CAD build for the part. Positions are in the model's coordinates, mm. A direction names the side the tool comes from. Give positions to 0.01 mm unless a question says otherwise; leave off trailing zeros. Loops run counter-clockwise (first coordinate to the right, second up) from the corner with the lowest first, then second, coordinate; pieces in that order, holes last.
```python
from build123d import *

# Parameters (mm, degrees)
BOSS_EXTRUDE1_DEPTH       = 3.175
SKETCH2_R                 = 3.302
BOSS_EXTRUDE2_DEPTH       = 3.175
BOSS_EXTRUDE3_DEPTH       = 3.175
BOSS_EXTRUDE4_DEPTH       = 3.175
SKETCH10_R                = 3.302
CUT_EXTRUDE2_DEPTH        = 3.175
BOSS_EXTRUDE6_DEPTH       = 3.175
F_6_CLEARANCE_HOLE1_D     = 3.7973
F_6_CLEARANCE_HOLE1_DEPTH = 25.4
F_6_CLEARANCE_HOLE1_TIP   = 1.140824014
CUT_EXTRUDE8_DEPTH        = 4.7625
SKETCH4_R                 = 25.4
BOSS_EXTRUDE7_DEPTH       = 3.175
CUT_EXTRUDE9_DEPTH        = 3.175
SKETCH19_R                = 9.525
CUT_EXTRUDE10_DEPTH       = 3.175
CUT_EXTRUDE12_DEPTH       = 4.175


with BuildPart() as part:
    # Sketch1 → Boss-Extrude1 (new body)
    with BuildSketch(Plane.XY):
        Polygon((-150.669615327, -62.417005507), (-62.404018861, -150.674994572), (62.417005507, -150.669615327), (150.674994572, -62.404018861), (150.669615327, 62.417005507), (62.404018861, 150.674994572), (-62.417005507, 150.669615327), (-150.674994572, 62.404018861), align=None)
        Polygon((-137.969842044, -57.155945955), (-57.144053939, -137.974767879), (57.155945955, -137.969842044), (137.974767879, -57.144053939), (137.969842044, 57.155945955), (57.144053939, 137.974767879), (-57.155945955, 137.969842044), (-137.974767879, 57.144053939), align=None, mode=Mode.SUBTRACT)
    extrude(amount=BOSS_EXTRUDE1_DEPTH)

    # Sketch2 → Boss-Extrude2 (add)
    with BuildSketch(Plane.XY.offset(3.175)):
        with BuildLine():
            Line((-104.300258744, 90.821465649), (-90.83045509, 104.292430334))
            ThreePointArc((-90.83045509, 104.292430334), (-90.829874575, 90.822046164), (-104.300258744, 90.821465649))
        make_face()
        with Locations((-94.197615746, 94.189497078)):
            Circle(SKETCH2_R, mode=Mode.SUBTRACT)
        with BuildLine():
            Line((104.292430334, 90.83045509), (90.821465649, 104.300258744))
            ThreePointArc((90.821465649, 104.300258744), (90.822046164, 90.829874575), (104.292430334, 90.83045509))
        make_face()
        with Locations((94.189497078, 94.197615746)):
            Circle(SKETCH2_R, mode=Mode.SUBTRACT)
        with BuildLine():
            Line((104.300258744, -90.821465649), (90.83045509, -104.292430334))
            ThreePointArc((90.83045509, -104.292430334), (90.829874575, -90.822046164), (104.300258744, -90.821465649))
        make_face()
        with Locations((94.197615746, -94.189497078)):
            Circle(SKETCH2_R, mode=Mode.SUBTRACT)
        with BuildLine():
            Line((-104.292430334, -90.83045509), (-90.821465649, -104.300258744))
            ThreePointArc((-90.821465649, -104.300258744), (-90.822046164, -90.829874575), (-104.292430334, -90.83045509))
        make_face()
        with Locations((-94.189497078, -94.197615746)):
            Circle(SKETCH2_R, mode=Mode.SUBTRACT)
    extrude(amount=-BOSS_EXTRUDE2_DEPTH)

    # Sketch5 → Boss-Extrude3 (add)
    with BuildSketch(Plane.XY.offset(3.175)):
        with BuildLine():
            Line((137.970389359, 44.455945967), (137.969842044, 57.155945955))
            Line((137.969842044, 57.155945955), (128.989198921, 66.135815058))
            ThreePointArc((128.989198921, 66.135815058), (126.236781441, 52.295360716), (137.970389359, 44.455945967))
        make_face()
        with BuildLine():
            Line((128.994898776, -66.124697061), (137.974767879, -57.144053939))
            Line((137.974767879, -57.144053939), (137.974220564, -44.44405395))
            ThreePointArc((137.974220564, -44.44405395), (126.241288378, -52.284480005), (128.994898776, -66.124697061))
        make_face()
        with BuildLine():
            Line((-137.969842044, -57.155945955), (-137.970389359, -44.455945967))
            ThreePointArc((-137.970389359, -44.455945967), (-126.236781441, -52.295360716), (-128.989198921, -66.135815058))
            Line((-128.989198921, -66.135815058), (-137.969842044, -57.155945955))
        make_face()
        with BuildLine():
            Line((-137.974220564, 44.44405395), (-137.974767879, 57.144053939))
            Line((-137.974767879, 57.144053939), (-128.994898776, 66.124697061))
            ThreePointArc((-128.994898776, 66.124697061), (-126.241288378, 52.284480005), (-137.974220564, 44.44405395))
        make_face()
    extrude(amount=-BOSS_EXTRUDE3_DEPTH)

    # Sketch9 → Boss-Extrude4 (add)
    with BuildSketch(Plane(origin=(0, 0, 0), x_dir=(-1, 0, 0), z_dir=(0, 0, -1))):
        Polygon((-57.144053939, 137.974767879), (-137.969842044, 57.155945955), (-137.974767879, -57.144053939), (-57.155945955, -137.969842044), (57.144053939, -137.974767879), (137.969842044, -57.155945955), (137.974767879, 57.144053939), (57.155945955, 137.969842044), align=None)
        Polygon((-49.254106555, 118.924427839), (-118.92018212, 49.264356627), (-118.924427839, -49.254106555), (-49.264356627, -118.92018212), (49.254106555, -118.924427839), (118.92018212, -49.264356627), (118.924427839, 49.254106555), (49.264356627, 118.92018212), align=None, mode=Mode.SUBTRACT)
    extrude(amount=-BOSS_EXTRUDE4_DEPTH)

    # Sketch10 → Cut-Extrude2 (cut)
    with BuildSketch(Plane.XY):
        with Locations((-94.197615746, 94.189497078)):
            Circle(SKETCH10_R)
        with Locations((94.189497078, 94.197615746)):
            Circle(SKETCH10_R)
        with Locations((-94.189497078, -94.197615746)):
            Circle(SKETCH10_R)
        with Locations((94.197615746, -94.189497078)):
            Circle(SKETCH10_R)
    extrude(amount=CUT_EXTRUDE2_DEPTH, mode=Mode.SUBTRACT)

    # Sketch12 → Boss-Extrude6 (add)
    with BuildSketch(Plane(origin=(0, 0, 0), x_dir=(-1, 0, 0), z_dir=(0, 0, -1))):
        Polygon((6.35, 150.672031572), (-6.35, 150.672031572), (-6.35, 6.35), (-150.672578887, 6.35), (-150.672578887, -6.35), (-6.35, -6.35), (-6.35, -150.672031572), (6.35, -150.672031572), (6.35, -6.35), (150.672578887, -6.35), (150.672578887, 6.35), (6.35, 6.35), align=None)
    extrude(amount=-BOSS_EXTRUDE6_DEPTH)

    # #6 Clearance Hole1
    with Locations(Plane(origin=(0, 0, 0), x_dir=(-1, 0, 0), z_dir=(0, 0, -1))):
        with Locations((-0.418811464, 60.325), (-0.418811464, -37.9222), (-0.418811464, -60.52312), (37.9222, 0), (60.52312, 0), (-60.325, 0)):
            Hole(F_6_CLEARANCE_HOLE1_D / 2, depth=F_6_CLEARANCE_HOLE1_DEPTH)
            with Locations((0, 0, -(F_6_CLEARANCE_HOLE1_DEPTH + F_6_CLEARANCE_HOLE1_TIP / 2))):  # 118° drill point
                Cone(0, F_6_CLEARANCE_HOLE1_D / 2, F_6_CLEARANCE_HOLE1_TIP, mode=Mode.SUBTRACT)

    # Sketch17 → Cut-Extrude8 (cut)
    with BuildSketch(Plane(origin=(0, 0, 0), x_dir=(-1, 0, 0), z_dir=(0, 0, -1))):
        Polygon((-73.383632924, 150.675467746), (-61.318869739, 134.799947792), (60.965361784, 134.794677872), (72.666366941, 150.669173624), align=None)
        Polygon((-61.147982987, -134.794670002), (61.136248536, -134.799939922), (73.018390518, -150.675452006), (-73.031609347, -150.669157884), align=None)
    extrude(amount=-CUT_EXTRUDE8_DEPTH, mode=Mode.SUBTRACT)

    # Sketch4 → Boss-Extrude7 (add)
    with BuildSketch(Plane.XY.offset(3.175)):
        Circle(SKETCH4_R)
    extrude(amount=-BOSS_EXTRUDE7_DEPTH)

    # Sketch18 → Cut-Extrude9 (cut)
    with BuildSketch(Plane.XY.offset(3.175)):
        with BuildLine():
            ThreePointArc((109.296804613, 81.790472735), (103.174175191, 89.389946316), (96.524263045, 96.532582958))
            ThreePointArc((96.524263045, 96.532582958), (91.854529866, 96.532381713), (91.854731111, 91.862648534))
            ThreePointArc((91.854731111, 91.862648534), (98.182941997, 85.065549572), (104.009378392, 77.833713966))
            ThreePointArc((104.009378392, 77.833713966), (108.631470887, 77.16838024), (109.296804613, 81.790472735))
        make_face()
        with BuildLine():
            ThreePointArc((81.790472735, -109.296804613), (89.389946316, -103.174175191), (96.532582958, -96.524263045))
            ThreePointArc((96.532582958, -96.524263045), (96.532381713, -91.854529866), (91.862648534, -91.854731111))
            ThreePointArc((91.862648534, -91.854731111), (85.065549572, -98.182941997), (77.833713966, -104.009378392))
            ThreePointArc((77.833713966, -104.009378392), (77.16838024, -108.631470887), (81.790472735, -109.296804613))
        make_face()
        with BuildLine():
            ThreePointArc((-109.296804613, -81.790472735), (-103.174175191, -89.389946316), (-96.524263045, -96.532582958))
            ThreePointArc((-96.524263045, -96.532582958), (-91.854529866, -96.532381713), (-91.854731111, -91.862648534))
            ThreePointArc((-91.854731111, -91.862648534), (-98.182941997, -85.065549572), (-104.009378392, -77.833713966))
            ThreePointArc((-104.009378392, -77.833713966), (-108.631470887, -77.16838024), (-109.296804613, -81.790472735))
        make_face()
        with BuildLine():
            ThreePointArc((-81.790472735, 109.296804613), (-89.389946316, 103.174175191), (-96.532582958, 96.524263045))
            ThreePointArc((-96.532582958, 96.524263045), (-96.532381713, 91.854529866), (-91.862648534, 91.854731111))
            ThreePointArc((-91.862648534, 91.854731111), (-85.065549572, 98.182941997), (-77.833713966, 104.009378392))
            ThreePointArc((-77.833713966, 104.009378392), (-77.16838024, 108.631470887), (-81.790472735, 109.296804613))
        make_face()
    extrude(amount=-CUT_EXTRUDE9_DEPTH, mode=Mode.SUBTRACT)

    # Sketch19 → Cut-Extrude10 (cut)
    with BuildSketch(Plane.XY.offset(3.175)):
        with Locations((-79.81209335, 106.653091503)):
            Circle(SKETCH19_R)
        with Locations((106.653091503, 79.81209335)):
            Circle(SKETCH19_R)
        with Locations((79.81209335, -106.653091503)):
            Circle(SKETCH19_R)
        with Locations((-106.653091503, -79.81209335)):
            Circle(SKETCH19_R)
    extrude(amount=-CUT_EXTRUDE10_DEPTH, mode=Mode.SUBTRACT)

    # Sketch22 → Cut-Extrude12 (cut, through all)
    with BuildSketch(Plane.XY.offset(3.175)):
        with BuildLine():
            Line((-137.97442785, 49.253969726), (-137.970182132, -49.264493456))
            ThreePointArc((-137.970182132, -49.264493456), (-134.795045306, -52.439356624), (-131.620182138, -49.264219798))
            Line((-131.620182138, -49.264219798), (-131.624427856, 49.254243384))
            ThreePointArc((-131.624427856, 49.254243384), (-134.799564682, 52.429106552), (-137.97442785, 49.253969726))
        make_face()
        with BuildLine():
            Line((131.869384327, 49.087223722), (131.740243733, -49.431154911))
            ThreePointArc((131.740243733, -49.431154911), (134.911079132, -52.610314057), (138.090238278, -49.439478658))
            Line((138.090238278, -49.439478658), (138.219378871, 49.078899975))
            ThreePointArc((138.219378871, 49.078899975), (135.048543473, 52.258059121), (131.869384327, 49.087223722))
        make_face()
    extrude(amount=-CUT_EXTRUDE12_DEPTH, mode=Mode.SUBTRACT)


solid = part.part
```
1. Saw through at A-A, the plane y = 80.5. List the corners of the cut face in (x, z) (3 decimals), and give its area (3 significant figures).
Responses:
outline: (-132.581, 0) - (-87.681, 0) - (-87.681, 3.175) - (-132.581, 3.175) - close; (-6.35, 0) - (6.35, 0) - (6.35, 3.175) - (-6.35, 3.175) - close; (87.682, 0) - (97.153, 0) - (97.153, 3.175) - (87.682, 3.175) - close; (116.153, 0) - (132.585, 0) - (132.585, 3.175) - (116.153, 3.175) - close
area: 265 mm2
2. Pull direction X, two halves, no side cores. Call faces 4 (the face through (92.7, -100.21, 1.61)), 5 (the face through (64.869, -139.765, 1.565)), 6 (the face through (110.23, 102.853, 1.565)): released by +X, released by -X, zero draft, split by the parting line, or undercut.
Responses:
face 4: undercut
face 5: undercut
face 6: released by +X
3. Probe line 1 along X through (y, z) = (-33, 1.3); line 2 along X through (y, z) = (-37.5, 0.9); line 3 along X through (y, z) = (-47.5, 1.7). List the from-to ranges inside material, lowest first.
Responses:
line 1: x = -150.67 to -137.97, -131.62 to -118.92, -6.35 to 6.35, 118.92 to 131.76, 138.11 to 150.67
line 2: x = -150.67 to -137.97, -131.62 to -118.92, -6.35 to -1.43, 2.27 to 6.35, 118.92 to 131.76, 138.11 to 150.67
line 3: x = -150.67 to -137.97, -131.62 to -118.92, -6.35 to 6.35, 118.92 to 131.74, 138.09 to 150.67
4. Saw through at B-B, the plane y = -81. List the corners of the cut face in (x, z) (3 decimals).
Responses:
outline: (-132.085, 0) - (-116.104, 0) - (-116.104, 3.175) - (-132.085, 3.175) - close; (-97.202, 0) - (-87.182, 0) - (-87.182, 3.175) - (-97.202, 3.175) - close; (-6.35, 0) - (6.35, 0) - (6.35, 3.175) - (-6.35, 3.175) - close; (87.181, 0) - (132.081, 0) - (132.081, 3.175) - (87.181, 3.175) - close
5. Drop flat-ended pins along their axis: pin 1 (1 mm diameter, centred on x = -26.5, z = 1.5, fed in from -Y); pin 2 (25 mm diameter, centred on x = 106.65, y = 79.81, fed in from +Z) (3 decimals); pin 3 (1.6 mm diameter, centred on y = -1.5, z = 1, fed in from +X); pin 4 (1.6 mm diameter, centred on y = 2, z = 1, fed in from -X). Give the stop position or say it passes through.
Responses:
pin 1: stops at y = -134.8
pin 2: stops at z = 3.175
pin 3: stops at x = 150.67
pin 4: stops at x = -150.67
6. Saw through at C-C, the plane x = 125. List the corners of the cut face in (y, z) (3 decimals), and give its area (3 significant figures).
Responses:
outline: (-88.081, 0) - (88.084, 0) - (88.084, 3.175) - (-88.081, 3.175) - close
area: 559 mm2
7. Saw through at D-D, the plane z = 1.5. Count the separate pieces of the cut face and the enclosed holes in it, and give its area (3 significant figures).
Responses:
separate pieces: 1
enclosed holes: 16
area: 28,200 mm2
8. Tool access for faces 1 (the face through (-84.58, 83.6, 1.57)), 2 (the face through (-64.59, 139.71, 1.57)), 3 (the face through (-64.75, -139.63, 1.57)): list every direction of +Z, -Z, +X, -X, +Y, -Y with a clear straight run to the whole face (end or side of a thin tool).
Responses:
face 1: +Z, -Z
face 2: +Z, -Z, +Y
face 3: +Z, -Z, -Y
